Input: part model. Units: mm. Frame: model coordinates. Give positions to 0.01 mm unless a question says otherwise; leave off trailing zeros. Write each loop counter-clockwise with the first axis right and the second up, starting at its lowest first coordinate (ties: lowest second). Pieces come first, ordered by that corner, then holes.
Autodesk Inventor part; units mm, degrees
ref_plane "YZ Plane" through (0, 0, 0) normal (1, 0, 0) x (0, 1, 0)
ref_plane "XZ Plane" through (0, 0, 0) normal (0, 1, 0) x (-1, 0, 0)
ref_plane "XY Plane" through (0, 0, 0) normal (0, 0, 1) x (1, 0, 0)
sketch "Skizze1" plane through (0, 0, 0) normal (1, 0, 0) x (0, 1, 0)
  line L0 (78.5, 96) -> (-78.5, 96)
  line L1 (-78.5, 96) -> (-78.5, -96)
  line L2 (-78.5, -96) -> (78.5, -96)
  line L3 (78.5, -96) -> (78.5, 96)
  point P0 (0, 0)
  dimension "d0" = 192
  dimension "d1" = 157
  dimension "d2" = 78.5
  dimension "d3" = 96
extrude "Extrusion1" add sketch "Skizze1" along normal blind 10
sketch "草图5" plane through (0, 0, 0) normal (-1, 0, 0) x (0, 0, 1)
  point P0 (0, 0)
sketch "草图6" plane through (10, 0, 0) normal (1, 0, 0) x (0, 0, -1)
  line L0 (-24, 25) -> (-72, 25)
  line L1 (-72, 25) -> (-72, -25)
  line L2 (-72, -25) -> (-24, -25)
  line L3 (-24, -25) -> (-24, 25)
  line L4 (-24, 25) -> (-72, -25) construction
  line L5 (-72, 25) -> (-24, -25) construction
  line L6 (-96, 78.5) -> (-96, -78.5)
  line L7 (-65.5, -17.5) -> (-30.5, -17.5)
  line L8 (-30.5, -17.5) -> (-30.5, 17.5)
  line L9 (-30.5, 17.5) -> (-65.5, 17.5)
  line L10 (-65.5, 17.5) -> (-65.5, -17.5)
  line L11 (-65.5, -17.5) -> (-30.5, 17.5) construction
  line L12 (-30.5, -17.5) -> (-65.5, 17.5) construction
  circle A0 centre (-65.5, -17.5) radius 2.5
  circle A1 centre (-30.5, -17.5) radius 2.5
  circle A2 centre (-30.5, 17.5) radius 2.5
  circle A3 centre (-65.5, 17.5) radius 2.5
  line L13 (24, 25) -> (72, 25)
  line L14 (72, 25) -> (72, -25)
  line L15 (72, -25) -> (24, -25)
  line L16 (24, -25) -> (24, 25)
  line L17 (24, 25) -> (72, -25) construction
  line L18 (72, 25) -> (24, -25) construction
  line L19 (65.5, -17.5) -> (30.5, -17.5)
  line L20 (30.5, -17.5) -> (30.5, 17.5)
  line L21 (30.5, 17.5) -> (65.5, 17.5)
  line L22 (65.5, 17.5) -> (65.5, -17.5)
  line L23 (65.5, -17.5) -> (30.5, 17.5) construction
  line L24 (30.5, -17.5) -> (65.5, 17.5) construction
  circle A4 centre (65.5, -17.5) radius 2.5
  circle A5 centre (30.5, -17.5) radius 2.5
  circle A6 centre (30.5, 17.5) radius 2.5
  circle A7 centre (65.5, 17.5) radius 2.5
  point P0 (0, 0)
  point P1 (-48, 0)
  point P2 (-48, 0)
  point P3 (48, 0)
  point P4 (48, 0)
  dimension "d31" = 50
  dimension "d32" = 48
  dimension "d33" = 24
  dimension "d34" = 35
  dimension "d35" = 35
  dimension "d36" = 5
  dimension "d39" = 360
  dimension "d48" = 5
  dimension "d49" = 5
  dimension "d50" = 5
  dimension "d51" = 5
hole "孔1" at (10, -17.5, 65.5) at (10, 17.5, 65.5) at (10, -17.5, 30.5) at (10, -17.5, -30.5) at (10, 17.5, -30.5) at (10, 17.5, -65.5) at (10, -17.5, -65.5) at (10, 17.5, 30.5) direction (-1, 0, 0) diameter 6 end through all
chamfer "倒角1" distance 0.5 angle 45 7 edges at (10, -17.5, -62.5) (10, 17.5, 33.5) (10, -17.5, 33.5) (10, -17.5, 68.5) (10, 17.5, -27.5) (10, -17.5, -27.5) (10, 17.5, -62.5)
sketch "草图7" plane through (10, 0, 0) normal (1, 0, 0) x (0, 0, -1)
  circle A0 centre (0, 0) radius 3.4
  circle A1 centre (30.5, 17.5) radius 3
  circle A2 centre (65.5, -17.5) radius 3.5
  line L0 (30.5, 17.5) -> (65.5, -17.5)
  circle A3 centre (65.5, 17.5) radius 3
  line L1 (65.5, 17.5) -> (30.5, -17.5)
  circle A4 centre (48, 0) radius 3.4
  circle A5 centre (-65.5, 17.5) radius 2.4585
  circle A6 centre (-30.5, -17.5) radius 3
  line L2 (-65.5, 17.5) -> (-30.5, -17.5)
  circle A7 centre (-30.5, 17.5) radius 3
  line L3 (-30.5, 17.5) -> (-65.5, -17.5)
  circle A8 centre (-48, 0) radius 3.4
  line L4 (48, 0) -> (48, 35)
  line L5 (37, 0) -> (59, 0)
  line L6 (43, 30) -> (54, 30)
  circle A9 centre (48, 25) radius 2.15
  line L7 (48, 0) -> (48, -21)
  circle A10 centre (48, -26.3861) radius 2.15
  line L8 (43, -25.3) -> (55, -25.3)
  line L9 (48, -20) -> (48, -32)
  dimension "d58" = 6.8
  dimension "d59" = 6.8
  dimension "d60" = 6.8
  dimension "d89" = 30
  dimension "d90" = 4.3
  dimension "d95" = 25.3
extrude "拉伸4" cut sketch "草图7" against normal blind 10 contours A0 | A4 L4 L0 | L0 L5 A4 | L5 A4 L0 | L4 A4 L1 | L7 A4 L1 | L1 A4 L5 | L1 A4 L5 | L0 A4 L7 | A8 L3 L2 | L2 L3 A8 | L3 A8 L2 | L2 A8 L3 | A9 L4 | L4 A9 | A10 L9 L8 | L8 L9 A10 | A10 L8 L9 | L9 L8 A10
chamfer "倒角3" distance 0.5 angle 45 3 edges at (10, 0, 51.4) (10, 0, 3.4) (10, 0, -44.6)
thread "螺纹3"
thread "螺纹4"
thread "螺纹5"
sketch "草图8" plane through (10, 0, 0) normal (1, 0, 0) x (0, 0, -1)
  line L0 (-87.5, 62.5) -> (87.5, 62.5)
  line L1 (87.5, 62.5) -> (87.5, -62.5)
  line L2 (87.5, -62.5) -> (-87.5, -62.5)
  line L3 (-87.5, -62.5) -> (-87.5, 62.5)
  circle A0 centre (0, 0) radius 3.9
  line L4 (-87.5, 62.5) -> (87.5, -62.5) construction
  line L5 (87.5, 62.5) -> (-87.5, -62.5) construction
  circle A1 centre (-87.5, 62.5) radius 3.25
  line L6 (-152, 0) -> (160, 0)
  line L7 (0, 94) -> (0, -105)
  circle A2 centre (-87.5, -62.5) radius 3.25
  circle A3 centre (87.5, 62.5) radius 3.25
  circle A4 centre (87.5, -62.5) radius 3.25
  dimension "d72" = 175
  dimension "d73" = 125
  dimension "d74" = 6.5
extrude "拉伸5" cut sketch "草图8" against normal blind 10 contours L3 A1 L0 | L0 A1 L3 | A3 L1 L0 | L0 L1 A3 | A2 L2 L3 | L3 L2 A2 | A4 L2 L1 | L1 L2 A4
chamfer "倒角4" distance 0.2 angle 45 4 edges at (10, 62.5, 90.75) (10, 62.5, -84.25) (10, -62.5, -84.25) (10, -62.5, 90.75)
thread "螺纹6"
thread "螺纹7"
thread "螺纹8"
thread "螺纹9"
thread "螺纹10"
thread "螺纹11"
properties part number "Adapterplatte_messstage_Gong_2025-03-28v00r00grm"
Q1. Section C-C, the plane z = 48. Return the cut outline in (x, y), then the cut area to 3 significant figures.
Q2. Pin query (flat end, axial travel): pin 1 (3.5 mm diameter, centred on y = 17.5, z = -65.5, fed in from +X). Return the tip coordinate at first contact, or that it passes through.
Q3. Section A-A, the plane z = -65.5. Return the cut outline in (x, y), then the cut area to 3 significant figures.
Q4. Mould query, pull axis Z, two halves, no side actions, for faces 1 (the flat face through (5, 1, 96)), 2 (the flat face through (5, 78.5, -1)), 3 (the cylindrical face through (4.82, -1.3, -51.14)). Classes: +Z half, -Z half, draft (parallel to the pull), parting line (faces both ways), or undercut.
Q5. Section D-D, the plane y = 25. Return the cut outline in (x, z).
Q6. Material intervals for line 1 along Z through (x, y) = (2.25, -17.5); line 2 along Z through (x, y) = (5.25, -62.5); line 3 along Y through (x, z) = (4.75, -48), sorted ascending.
Q7. Section B-B, the plane y = -62.5. Return the cut outline in (x, z).
Solutions:
1. outline: (0, -78.5) - (10, -78.5) - (10, -3.9) - (9.5, -3.4) - (0, -3.4) - close; (0, 3.4) - (9.5, 3.4) - (10, 3.9) - (10, 78.5) - (0, 78.5) - close
1. area: 1,500 mm2
2. pin 1: passes through
3. outline: (0, -78.5) - (10, -78.5) - (10, -21) - (9.5, -20.5) - (0, -20.5) - close; (0, -14.5) - (9.5, -14.5) - (10, -14) - (10, 14) - (9.5, 14.5) - (0, 14.5) - close; (0, 20.5) - (9.5, 20.5) - (10, 21) - (10, 78.5) - (0, 78.5) - close
3. area: 1,450 mm2
4. face 1: +Z half
4. face 2: draft
4. face 3: undercut
5. outline: (0, -96) - (10, -96) - (10, -50.15) - (0, -50.15) - close; (0, -45.85) - (10, -45.85) - (10, 96) - (0, 96) - close
6. line 1: z = -96 to -68.5, -62.5 to -33.5, -27.5 to 27.5, 33.5 to 62.5, 68.5 to 96
6. line 2: z = -96 to -90.75, -84.25 to 84.25, 90.75 to 96
6. line 3: y = -78.5 to -28.54, -24.24 to -3.4, 3.4 to 22.85, 27.15 to 78.5
7. outline: (0, -96) - (10, -96) - (10, -90.95) - (9.8, -90.75) - (0, -90.75) - close; (0, -84.25) - (9.8, -84.25) - (10, -84.05) - (10, 84.05) - (9.8, 84.25) - (0, 84.25) - close; (0, 90.75) - (9.8, 90.75) - (10, 90.95) - (10, 96) - (0, 96) - close
